Autodesk Inventor part; units mm, degrees
ref_plane "nut_XY" through (0, 0, 0) normal (1, 0, 0) x (0, 0, -1)
ref_plane "nut_YZ" through (0, 0, 0) normal (0, 0, -1) x (0, 1, 0)
ref_plane "nut_ZX" through (0, 0, 0) normal (0, 1, 0) x (1, 0, 0)
sketch "Sketch_1" plane through (0, 0, 0) normal (0, 0, 1) x (1, 0, 0)
  arc A0 (-6.3, -4.6492) -> (-6.0809, -5.2739) centre (-5.3, -4.6492) ccw
  line L0 (-6.0809, -5.2739) -> (-4.6002, -7.1247)
  arc A1 (-4.6002, -7.1247) -> (-3.8194, -7.5) centre (-3.8194, -6.5) ccw
  line L1 (-3.8194, -7.5) -> (-1.8, -7.5)
  arc A2 (-1.8, -7.5) -> (-0.8, -6.5) centre (-1.8, -6.5) ccw
  line L2 (-0.8, -6.5) -> (-0.8, -3.9)
  line L3 (-0.8, -3.9) -> (0, -3.9)
  line L4 (0, -3.9) -> (0, 3.9)
  line L5 (0, 3.9) -> (-0.8, 3.9)
  line L6 (-0.8, 3.9) -> (-0.8, 6.5)
  arc A3 (-0.8, 6.5) -> (-1.8, 7.5) centre (-1.8, 6.5) ccw
  line L7 (-1.8, 7.5) -> (-3.8194, 7.5)
  arc A4 (-3.8194, 7.5) -> (-4.6002, 7.1247) centre (-3.8194, 6.5) ccw
  line L8 (-4.6002, 7.1247) -> (-6.0809, 5.2739)
  arc A5 (-6.0809, 5.2739) -> (-6.3, 4.6492) centre (-5.3, 4.6492) ccw
  line L9 (-6.3, 4.6492) -> (-6.3, -4.6492)
extrude "Extrusion1" add sketch "Sketch_1" along normal mid plane 14
sketch "Sketch_5" plane through (0, 0, 0) normal (0, 0, 1) x (1, 0, 0)
  line L0 (0, 0) -> (-6.3, 0)
  line L1 (-6.3, 0) -> (-6.3, 2)
  line L2 (-6.3, 2) -> (-5.921, 1.621)
  line L3 (-5.921, 1.621) -> (-0.379, 1.621)
  line L4 (-0.379, 1.621) -> (0, 2)
  line L5 (0, 2) -> (0, 0)
  line L6 (0, 0) -> (-6.3, 0)
revolve "Revolution1" cut sketch "Sketch_5" angle 360 about axis through (0, 0, 0) along (1, 0, 0)
thread "Thread1"
ref_plane "nut_XY" through (0, 0, 0) normal (1, 0, 0) x (0, 0, -1)
ref_plane "nut_YZ" through (0, 0, 0) normal (0, 0, -1) x (0, 1, 0)
ref_plane "nut_ZX" through (0, 0, 0) normal (0, 1, 0) x (1, 0, 0)
ref_plane "to_bolt_XY" through (-6.3, 0, 0) normal (1, 0, 0) x (0, 0, -1)
ref_plane "to_bolt_YZ" through (-6.3, 0, 0) normal (0, 0, -1) x (0, 1, 0)
ref_plane "to_bolt_ZX" through (-6.3, 0, 0) normal (0, 1, 0) x (1, 0, 0)
ref_plane "to_frames_XY" through (-0.8, 0, 0) normal (1, 0, 0) x (0, 0, -1)
ref_plane "to_frames_YZ" through (-0.8, 0, 0) normal (0, 0, -1) x (0, 1, 0)
ref_plane "to_frames_ZX" through (-0.8, 0, 0) normal (0, 1, 0) x (1, 0, 0)
properties part number "HNTT6-4" material "ステンレス鋼"
Source: CAD feature listing. Evaluate the final solid. Frame: model axes, mm. A direction names the side the tool comes from. Give positions to 0.01 mm unless a question says otherwise; leave off trailing zeros. Order: outer loops, then holes, each group sorted by start corner. A loop starts at its lowest first (then second) coordinate and runs counter-clockwise, first axis right, second up. Notation, with made-up numbers: (59.5, 32.5) -> (83.5, 32.5) arc R15 ccw to (83.5, 52.5) -> close; hole circle Ø11 at (-33.75, 45). An arc over 180 degrees is marked (long way). Use a Markdown table: item, result.
1) Section query D-D, the plane z = 2.5. Return the cut outline in (x, y).
Answer list:
| item | result |
|---|---|
| outline | (-6.3, -4.65) arc R1 ccw to (-6.08, -5.27) -> (-4.6, -7.12) arc R1 ccw to (-3.82, -7.5) -> (-1.8, -7.5) arc R1 ccw to (-0.8, -6.5) -> (-0.8, -3.9) -> (0, -3.9) -> (0, 3.9) -> (-0.8, 3.9) -> (-0.8, 6.5) arc R1 ccw to (-1.8, 7.5) -> (-3.82, 7.5) arc R1 ccw to (-4.6, 7.12) -> (-6.08, 5.27) arc R1 ccw to (-6.3, 4.65) -> close |
2) Section query B-B, the plane y = 0. Return the cut outline in (x, z).
Answer list:
| item | result |
|---|---|
| outline | (-6.3, -7) -> (0, -7) -> (0, -2) -> (-0.38, -1.62) -> (-5.92, -1.62) -> (-6.3, -2) -> close; (-6.3, 2) -> (-5.92, 1.62) -> (-0.38, 1.62) -> (0, 2) -> (0, 7) -> (-6.3, 7) -> close |
3) Reachability of faces 1 (the flat face through (-0.8, 5, 0)), 2 (the flat face through (-0.8, -5, 0)), 3 (the flat face through (-5.35, -6.19, -0.1)) from +Z, -Z, +X, -X, +Y, -Y: full face, straight path, thin tool, end or side. Return the list, or none.
Answer list:
| item | result |
|---|---|
| face 1 | +Z, -Z, +X, +Y |
| face 2 | +Z, -Z, +X, -Y |
| face 3 | +Z, -Z, -X, -Y |
4) Section query C-C, the plane x = -3.25. Return the cut outline in (y, z), then the cut area to 3 significant figures.
Answer list:
| item | result |
|---|---|
| outline | (-7.5, -7) -> (7.5, -7) -> (7.5, 7) -> (-7.5, 7) -> close; hole circle Ø3.24 at (0, 0) |
| area | 202 mm² |
5) Mould query, pull axis Y, two halves, no side actions, for faces 4 (the flat face through (-3, 0, -7)), 5 (the cylindrical face through (-3.111, 0.748, -1.438)), 6 (the flat face through (-5.33, 6.21, -0.1)), 7 (the cylindrical face through (-1.085, -7.199, -0.098)). Classes: +Y half, -Y half, draft (parallel to the pull), parting line (faces both ways), or undercut.
Answer list:
| item | result |
|---|---|
| face 4 | draft |
| face 5 | undercut |
| face 6 | +Y half |
| face 7 | -Y half |
6) Section query A-A, the plane z = 0. Return the cut outline in (x, y), then the cut area to 3 significant figures.
Answer list:
| item | result |
|---|---|
| outline | (-6.3, -4.65) arc R1 ccw to (-6.08, -5.27) -> (-4.6, -7.12) arc R1 ccw to (-3.82, -7.5) -> (-1.8, -7.5) arc R1 ccw to (-0.8, -6.5) -> (-0.8, -3.9) -> (0, -3.9) -> (0, -2) -> (-0.38, -1.62) -> (-5.92, -1.62) -> (-6.3, -2) -> close; (-6.3, 2) -> (-5.92, 1.62) -> (-0.38, 1.62) -> (0, 2) -> (0, 3.9) -> (-0.8, 3.9) -> (-0.8, 6.5) arc R1 ccw to (-1.8, 7.5) -> (-3.82, 7.5) arc R1 ccw to (-4.6, 7.12) -> (-6.08, 5.27) arc R1 ccw to (-6.3, 4.65) -> close |
| area | 62.5 mm² |
7) Ray query, line 1 along Z through (x, y) = (-2.1, 0); line 2 along Y through (x, z) = (-5.5, -0.5); line 3 along Y through (x, z) = (-5.5, 0.25). Return the intervals inside material, ascending. Write a range as [from, to].
Answer list:
| item | result |
|---|---|
| line 1 | [-7, -1.62], [1.62, 7] |
| line 2 | [-6, -1.54], [1.54, 6] |
| line 3 | [-6, -1.6], [1.6, 6] |
8) Contact query for flat-ended pins moving along their axis: P1, Ø1.3, axis at y = -5.5, z = -0.5, coming from the +X side; P2, Ø0.6, axis at x = 0, z = 0, coming from the +Y side. Output: stop coordinate, or through.
Answer list:
| item | result |
|---|---|
| P1 | x = -0.8 |
| P2 | y = 3.9 |
